Work out the finished part from the listing and answer in its coordinate system (mm). A direction names the side the tool comes from. Coordinates: 2 decimals unless noted, no trailing zeros. Write each loop counter-clockwise with the first axis right and the second up, starting at its lowest first coordinate (ties: lowest second). Pieces come first, ordered by that corner, then holes. Notation, with made-up numbers: M 66,68.5 L 82,68.5 A21 cw 82,103.5 Z; hole C 28,85 d2. An arc over 180 degrees is marked long. Answer as CSV lines item,"result". Start each with the question number.
(1) Flat-ended cylindrical pins translate along their axes: P1, Ø1.1, axis at y = 1, z = -30, coming from the -X side; P2, Ø4, axis at x = 39.5, z = -12.5, coming from the -Y side; P3, Ø4.5, axis at x = 18.161, z = -41.402, coming from the +Y side. Find the tip coordinate at first contact, or state that the pin passes through.
(2) A cutting plane is placed at D-D on z = -11.5. Give the vertices of the cut face in (x, y) (3 decimals), then the cut area to 3 significant figures.
(3) Find the intervals of material crossed by L1, parallel to Z at x = 18.5, y = 0.5; L2, parallel to Y at x = 19, z = -33; L3, parallel to X at y = 1.55, z = -29.5, in increasing order. Write a range as [from, to].
(4) A cutting plane is placed at A-A on x = 11. Give the vertices of the cut face in (y, z).
(5) A cutting plane is placed at C-C on y = 0.3. Give the vertices of the cut face in (x, z).
(6) A cutting plane is placed at B-B on z = -31. Give the vertices of the cut face in (x, y) (3 decimals), then the cut area to 3 significant figures.
(7) The mould has two halves that part along X. Classify faces 4 (the cylindrical face through (18.22, 0.69, -42.73)), 5 (the cylindrical face through (10.34, 0.69, -5.17)), 6 (the flat face through (38, 1, 0)), 7 (the flat face through (76.2, 1, -23)): released by +X, released by -X, zero draft, split by the parting line, or undercut.
(8) For faces 1 (the flat face through (17, 1.397, -18)), 2 (the flat face through (46, 0, -23)), 3 (the flat face through (8, 1, -15.24)), determine the directions among +Z, -Z, +X, -X, +Y, -Y from which every point of the face is accessible in a straight line to the end or side of a thin tool.
from build123d import *

# Parameters (mm, degrees)
SKETCH1_R           = 2.159
SKETCH1_R_2         = 1.330733042
BOSS_EXTRUDE1_DEPTH = 1.397
SKETCH1_3_W         = 52.448824391
SKETCH1_3_H         = 46.101
BOSS_EXTRUDE2_DEPTH = 1.905


with BuildPart() as part:
    # Sketch1 → Boss-Extrude1 (new body)
    with BuildSketch(Plane(origin=(0, 0, 0), x_dir=(1, 0, 0), z_dir=(0, 1, 0))):
        Polygon((0, 15.24), (0, 0), (76.2, 0), (76.2, 46.101), (15.24, 46.101), (15.24, 15.24), align=None)
        with Locations(Location((12.446, 4.699, 0), (0, 0, 270))):
            Circle(SKETCH1_R, mode=Mode.SUBTRACT)
        with Locations(Location((18.161, 4.699, 0), (0, 0, 270))):
            Circle(SKETCH1_R_2, mode=Mode.SUBTRACT)
        with Locations(Location((18.161, 41.402, 0), (0, 0, 270))):
            Circle(SKETCH1_R_2, mode=Mode.SUBTRACT)
    extrude(amount=BOSS_EXTRUDE1_DEPTH)

    # Sketch1_3 → Boss-Extrude2 (add)
    with BuildSketch(Plane(origin=(0, 0, 0), x_dir=(1, 0, 0), z_dir=(0, 1, 0))):
        with Locations((49.975587805, 23.0505)):
            Rectangle(SKETCH1_3_W, SKETCH1_3_H)
    extrude(amount=BOSS_EXTRUDE2_DEPTH)


solid = part.part
Here are the results:
1,P1,"stops at x = 15.24"
1,P2,"stops at y = 0"
1,P3,"stops at y = 1.4"
2,outline,"M 0,0 L 76.2,0 L 76.2,1.905 L 23.751,1.905 L 23.751,1.397 L 0,1.397 Z"
2,area,"133 mm^2"
3,L1,"z = [-46.1, -42.69], [-40.12, -5.99], [-3.41, 0]"
3,L2,"y = [0, 1.4]"
3,L3,"x = [23.75, 76.2]"
4,outline,"M 0,-15.24 L 1.4,-15.24 L 1.4,-6.3 L 0,-6.3 Z; M 0,-3.1 L 1.4,-3.1 L 1.4,0 L 0,0 Z"
5,outline,"M 0,-15.24 L 15.24,-15.24 L 15.24,-46.1 L 76.2,-46.1 L 76.2,0 L 0,0 Z; hole C 12.45,-4.7 d4.32; hole C 18.16,-41.4 d2.66; hole C 18.16,-4.7 d2.66"
6,outline,"M 15.24,0 L 76.2,0 L 76.2,1.905 L 23.751,1.905 L 23.751,1.397 L 15.24,1.397 Z"
6,area,"112 mm^2"
7,face 4,"undercut"
7,face 5,"undercut"
7,face 6,"zero draft"
7,face 7,"released by +X"
8,face 1,"+Z, -Z, -X, +Y"
8,face 2,"+Z, -Z, +X, -X, -Y"
8,face 3,"-Z, -X, +Y, -Y"
